```python
from build123d import *

# Parameters (mm, degrees)
F0_R     = 12.5
F1_DEPTH = 50
F2_R     = 12.5
F3_DEPTH = 25
F4_R     = 10
F5_DEPTH = 50.001
F6_R     = 10
F7_DEPTH = 25
F8_R     = 2


with BuildPart() as f1:
    # F0 (on Top) → F1 (new body)
    with BuildSketch(Plane.XY):
        Circle(F0_R)
    extrude(amount=F1_DEPTH)

    # F2 (on Front) → F3 (join)
    with BuildSketch(Plane.XZ):
        with Locations((0, 25)):
            Circle(F2_R)
    extrude(amount=F3_DEPTH)

    # F4 (on face) → F5 (cut, through all)
    with BuildSketch(Plane(origin=(0, 0, 0), x_dir=(1, 0, 0), z_dir=(0, 0, -1))):
        Circle(F4_R)
    extrude(amount=-F5_DEPTH, mode=Mode.SUBTRACT)

    # F6 (on face) → F7 (cut)
    with BuildSketch(Plane.XZ.offset(25)):
        with Locations((0, 25)):
            Circle(F6_R)
    extrude(amount=-F7_DEPTH, mode=Mode.SUBTRACT)

    # F8
    f8_edges = [f1.edges().sort_by_distance(p)[0] for p in [
        (9.5412, -8.075611, 16.924389),
        (-9.5412, -8.075611, 16.924389),
        (-1.4e-05, -12.5, 37.5),
    ]]
    fillet(f8_edges, radius=F8_R)


solid = f1.part
```
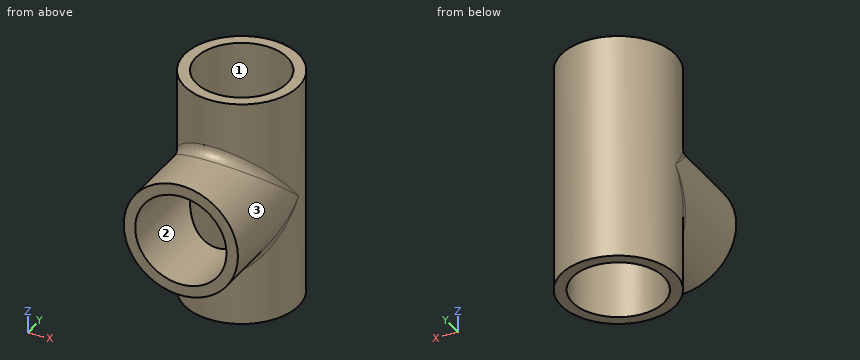
Input: part model. Units: mm. Frame: model coordinates. Face numbers are marked on the shaded views. Round coordinates to 2 decimals unless told otherwise and drop trailing zeros. Write each loop counter-clockwise with the first axis right and the second up, starting at its lowest first coordinate (ties: lowest second). Pieces come first, ordered by that corner, then holes. Notation, with made-up numbers: (45.25, 55.25) - (92.25, 55.25) arc R22 ccw to (92.25, 64.25) - close; hole circle Ø7 at (-2.75, 48.5). An arc over 180 degrees is marked (long way). Write item = value, one per line.
(1) Section query B-B on z = 9. Output: boundary loops of the cut face in (x, y).
Geometry check:
outline = circle Ø25 at (0, 0); hole circle Ø20 at (0, 0)
(2) Section query A-A on x = 0. State how many separate pieces and enclosed holes the cut face has, then the cut area to 3 significant figures.
Geometry check:
separate_pieces = 3
enclosed_holes = 0
area = 264 mm^2
(3) Contact query for flat-ended pins moving along their axis: pin 1 Ø1.5 at (y, z) = (-8, 12) entering from +X; pin 2 Ø3 at (x, z) = (-3.5, 25.5) entering from -Y; pin 3 Ø3 at (x, z) = (-6, 33.5) entering from +Y. Output: stop coordinate, or through.
Geometry check:
pin_1 = 10.18
pin_2 = 8.66
pin_3 = 11.66
(4) Pull-direction query (Z, two-part tool) for the marked faces 1, 2 and 3; classes: +Z half, -Z half, draft (parallel to the pull), parting line (faces both ways), or undercut.
Geometry check:
face_1 = draft
face_2 = undercut
face_3 = parting line
(5) Material intervals for probe 1 along Y at (x, z) = (0, 8.5); probe 2 along Z at (x, y) = (-0.25, -14.5), sorted ascending.
Geometry check:
probe_1 = -12.5 to -10, 10 to 12.5
probe_2 = 12.5 to 15, 35 to 37.5
(6) Section query C-C on y = -18. Output: boundary loops of the cut face in (x, z).
Geometry check:
outline = circle Ø25 at (0, 25); hole circle Ø20 at (0, 25)
